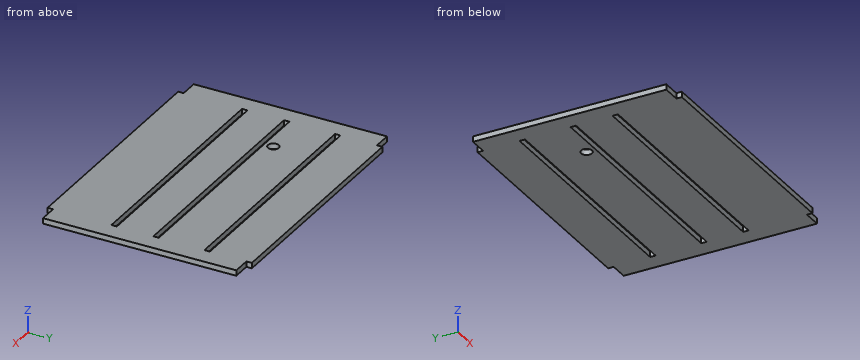
```python
from build123d import *

# Parameters (mm, degrees)
SKETCH1_W           = 130
SKETCH1_H           = 3
SKETCH1_R           = 3
BOSS_EXTRUDE1_DEPTH = 3


with BuildPart() as part:
    # Sketch1 → Boss-Extrude1 (new body)
    with BuildSketch(Plane.XY):
        Polygon((70.303030303, 34.481481481), (-59.696969697, 34.481481481), (-59.696969697, 31.481481481), (-69.696969697, 31.481481481), (-69.696969697, -74.518518519), (-59.696969697, -74.518518519), (-59.696969697, -77.518518519), (70.303030303, -77.518518519), (70.303030303, -74.518518519), (80.303030303, -74.518518519), (80.303030303, 31.481481481), (70.303030303, 31.481481481), align=None)
        with Locations((5.303030303, -41.018518519)):
            Rectangle(SKETCH1_W, SKETCH1_H, mode=Mode.SUBTRACT)
        with Locations((-34.696969697, -11.518518519)):
            Circle(SKETCH1_R, mode=Mode.SUBTRACT)
        with Locations((5.303030303, -18.018518519)):
            Rectangle(SKETCH1_W, SKETCH1_H, mode=Mode.SUBTRACT)
        with Locations((5.303030303, 9.981481481)):
            Rectangle(SKETCH1_W, SKETCH1_H, mode=Mode.SUBTRACT)
    extrude(amount=BOSS_EXTRUDE1_DEPTH)


solid = part.part
```
Input: part model. Units: mm. Frame: model coordinates. Round coordinates to 2 decimals unless told otherwise and drop trailing zeros. Order: outer loops, then holes, each group sorted by start corner. A loop starts at its lowest first (then second) coordinate and runs counter-clockwise, first axis right, second up. Notation, with made-up numbers: (66, 73.25) - (106, 73.25) arc R20 cw to (106, 83.25) - close; hole circle Ø3 at (66, -6.75). An arc over 180 degrees is marked (long way). One line per question, with ' | ' between items. Start each with the question number.
1) Ray query, probe 1 along Y at (x, z) = (-28, 2.7); probe 2 along Y at (x, z) = (-61, 0.75); probe 3 along X at (y, z) = (-17.5, 1.7). Return the intervals inside material, ascending.
2) Cut plane B-B, the plane z = 1.95. Return the cut outline in (x, y).
3) Contact query for flat-ended pins moving along their axis: P1, Ø0.9, axis at x = 75, z = 1.5, coming from the -Y side; P2, Ø12, axis at x = -47.5, y = 7.5, coming from the -Z side; P3, Ø1.5, axis at y = -75.5, z = 2, coming from the -X side; P4, Ø1.5, axis at y = 33, z = 1.5, coming from the +X side. Output: stop coordinate, or through.
4) Cut plane A-A, the plane x = 66. Return the cut outline in (y, z), then the cut area to 3 significant figures.
Worked out:
1) probe 1: y = -77.52 to -42.52, -39.52 to -19.52, -16.52 to 8.48, 11.48 to 34.48 | probe 2: y = -74.52 to 31.48 | probe 3: x = -69.7 to -59.7, 70.3 to 80.3
2) outline: (-69.7, -74.52) - (-59.7, -74.52) - (-59.7, -77.52) - (70.3, -77.52) - (70.3, -74.52) - (80.3, -74.52) - (80.3, 31.48) - (70.3, 31.48) - (70.3, 34.48) - (-59.7, 34.48) - (-59.7, 31.48) - (-69.7, 31.48) - close; hole (-59.7, -42.52) - (70.3, -42.52) - (70.3, -39.52) - (-59.7, -39.52) - close; hole (-59.7, -19.52) - (70.3, -19.52) - (70.3, -16.52) - (-59.7, -16.52) - close; hole (-59.7, 8.48) - (70.3, 8.48) - (70.3, 11.48) - (-59.7, 11.48) - close; hole circle Ø6 at (-34.7, -11.52)
3) P1: stops at y = -74.52 | P2: stops at z = 0 | P3: stops at x = -59.7 | P4: stops at x = 70.3
4) outline: (-77.52, 0) - (-42.52, 0) - (-42.52, 3) - (-77.52, 3) - close; (-39.52, 0) - (-19.52, 0) - (-19.52, 3) - (-39.52, 3) - close; (-16.52, 0) - (8.48, 0) - (8.48, 3) - (-16.52, 3) - close; (11.48, 0) - (34.48, 0) - (34.48, 3) - (11.48, 3) - close | area: 309 mm^2
